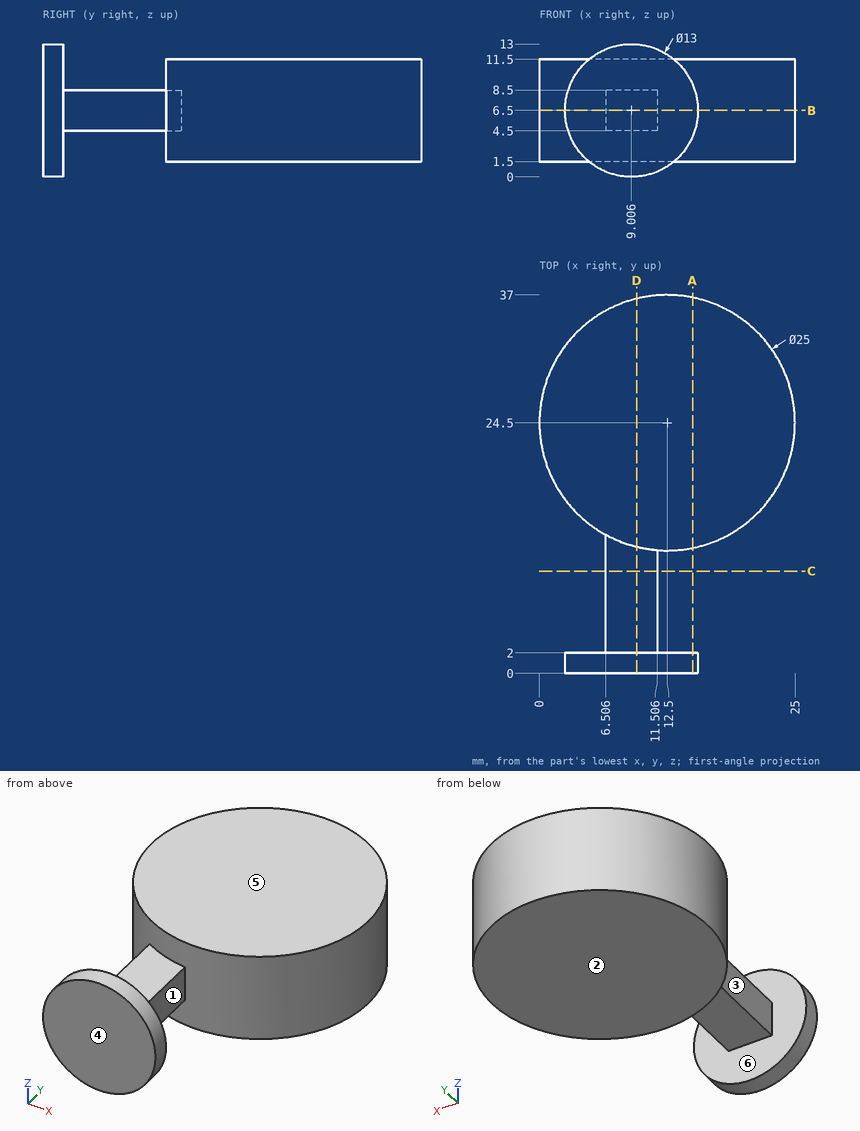
Could you check a few things on this drawing? It's one solid part, dimensions in mm from its lowest x, y, z. A direction names the side the tool comes from. Give positions to 0.01 mm unless a question says otherwise; leave off trailing zeros. Order: outer loops, then holes, each group sorted by start corner. A loop starts at its lowest first (then second) coordinate and runs counter-clockwise, first axis right, second up. Notation, with made-up numbers: (-25, -21) - (-4, -21) arc R22 cw to (-4, 7) - close; hole circle Ø7 at (62, 63.25). An arc over 180 degrees is marked (long way). One line per item, written item: value. Start each with the question number.
1. If I drill on probe 1 along Y at (x, z) = (12.25, 4); probe 2 along Z at (x, y) = (3.25, 21.5); probe 3 along Y at (x, z) = (14.5, 3.5), over which ranges is the centre line in solid material (lowest first)?
2. Imagine slicing it at D-D on x = 9.5. List the corners of the cut face in (y, z) for me (1 decimal), plus the area to 3 significant figures.
3. Thinking about a two-plate mould opening in Y: for the marked faces 1, 2, 3 and 4, which applies, +Y half, -Y half, draft (parallel to the pull), parting line (faces both ways), or undercut?
4. For P1, Ø12.5, axis at x = 7, y = 25.5, coming from the +Z side; P2, Ø4, axis at x = 9.5, z = 4.5, coming from the +Y side; P3, Ø1.2, axis at y = 9, z = 5.5, coming from the -X side, each with a flat end and sliding along its axis, tell me the tip position at first contact or that it passes through.
5. Imagine slicing it at B-B on z = 6.5. List the corners of the cut face in (x, y) for me, plus the area to 3 significant figures.
6. For the marked faces 5 and 6, which set-ups out of +Z, -Z, +X, -X, +Y, -Y let a thin tool reach every point of the face, with its end or its side?
7. Imagine slicing it at A-A on x = 15. List the corners of the cut face in (y, z) for me, plus the area to 3 significant figures.
8. Imagine slicing it at C-C on y = 10. List the corners of the cut face in (x, z) for me, plus the area to 3 significant figures.
Values:
1. probe 1: 0 to 2, 12 to 37
1. probe 2: 1.5 to 11.5
1. probe 3: 0 to 2, 12.16 to 36.84
2. outline: (0, 0) - (2, 0) - (2, 4.5) - (12.4, 4.5) - (12.4, 1.5) - (36.6, 1.5) - (36.6, 11.5) - (12.4, 11.5) - (12.4, 8.5) - (2, 8.5) - (2, 13) - (0, 13) - close
2. area: 310 mm²
3. face 1: undercut
3. face 2: draft
3. face 3: undercut
3. face 4: -Y half
4. P1: z = 11.5
4. P2: y = 36.96
4. P3: x = 6.51
5. outline: (2.51, 0) - (15.51, 0) - (15.51, 2) - (11.51, 2) - (11.51, 12.04) arc R12.5 ccw (long way) to (6.51, 13.53) - (6.51, 2) - (2.51, 2) - close
5. area: 570 mm²
6. face 5: +Z, +X, -X, +Y
6. face 6: none
7. outline: (0, 3.99) - (2, 3.99) - (2, 9.01) - (0, 9.01) - close; (12.25, 1.5) - (36.75, 1.5) - (36.75, 11.5) - (12.25, 11.5) - close
7. area: 255 mm²
8. outline: (6.51, 4.5) - (11.51, 4.5) - (11.51, 8.5) - (6.51, 8.5) - close
8. area: 20.0 mm²
